Part print with two shaded views. Sizes in mm from the minimum x, y, z corner. A direction names the side the tool comes from. Give positions to 0.01 mm unless a question says otherwise; leave off trailing zeros. Order: outer loops, then holes, each group sorted by start corner. A loop starts at its lowest first (then second) coordinate and runs counter-clockwise, first axis right, second up. Notation, with made-up numbers: (-7.5, 35.5) -> (38.5, 35.5) arc R19 cw to (38.5, 69.5) -> close; hole circle Ø8 at (4, 28). An arc over 180 degrees is marked (long way). Write item = value, one per line. Start each with the question number.
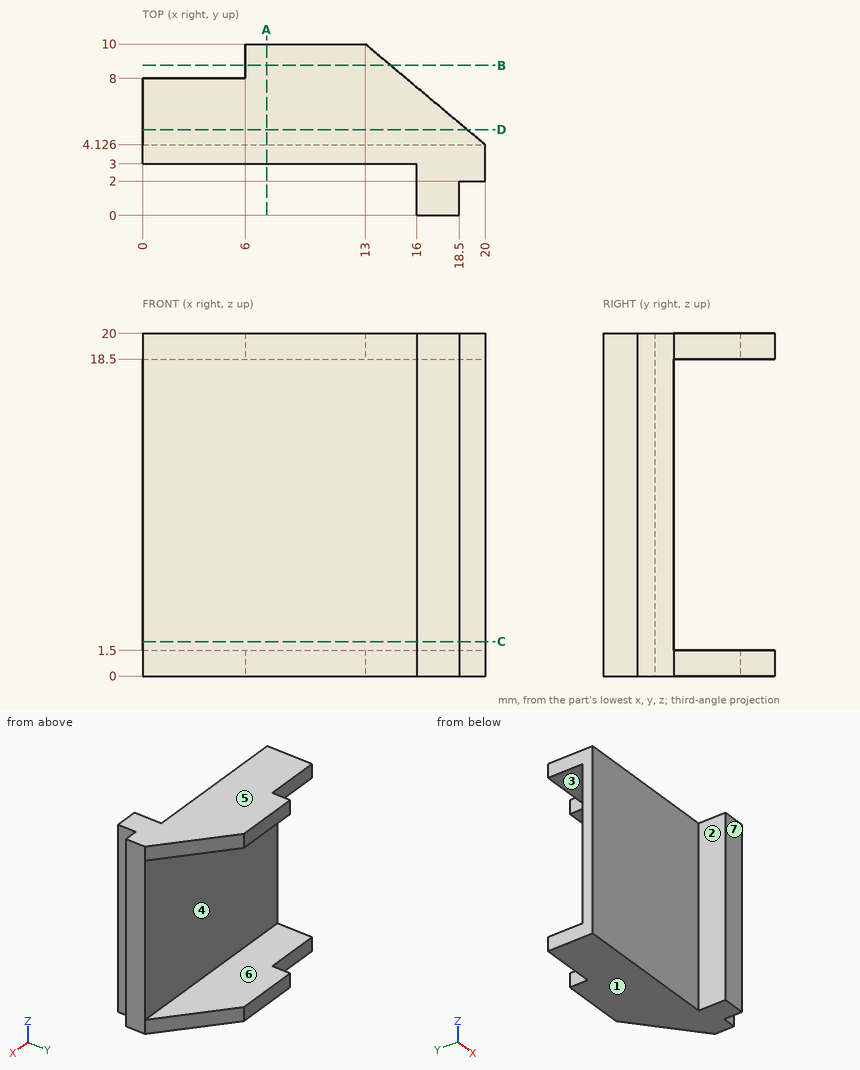
(1) Cut at C-C, the plane z = 2. Give the cut face in (x, y).
(2) 3-axis set-ups, long thin cutter, end or side, ignore diameter. For the marked faces 1, 2 and 3: which of +Z, -Z, +X, -X, +Y, -Y reach the whole face in a straight line?
(3) Cut at B-B, the plane y = 8.75. Give the cut face in (x, z).
(4) Flat gauge pins, fed straight in: P1, Ø0.8, axis at x = 19, z = 12.5, coming from the -Y side; P2, Ø2, axis at x = 13.5, z = 8.5, coming from the +Y side; P3, Ø3, axis at y = 8.5, z = 4.5, coming from the +X side; P4, Ø1.2, axis at y = 9, z = 19, coming from the -X side. Where does each tip first touch, or does it go through?
(5) Wall check: line 1 (Z direction, x = 8, y = 6.75); line 2 (Y direction, x = 4.5, z = 3.75); line 3 (X direction, y = 1, z = 15). Give the ranges that are in metal, low to high. Write a range as [from, to].
(6) Cut at A-A, the plane x = 7.25. Give the cut face in (y, z).
(7) Mould opens along Z. For the marked faces 4, 5, 6 and 7 say: released by +Z, released by -Z, zero draft, split by the parting line, or undercut.
(8) Cut at D-D, the plane y = 5. Give the cut face in (x, z).
Results:
q1.outline = (0, 3) -> (16, 3) -> (16, 0) -> (18.5, 0) -> (18.5, 2) -> (20, 2) -> (20, 4.13) -> (0, 4.13) -> close
q2.face_1 = -Z, +X, -X, +Y, -Y
q2.face_2 = +Z, -Z, -X, -Y
q2.face_3 = +X, -X, +Y
q3.outline = (6, 0) -> (14.49, 0) -> (14.49, 1.5) -> (6, 1.5) -> close; (6, 18.5) -> (14.49, 18.5) -> (14.49, 20) -> (6, 20) -> close
q4.P1 = 2
q4.P2 = 4.13
q4.P3 = through
q4.P4 = 6
q5.line_1 = [0, 1.5], [18.5, 20]
q5.line_2 = [3, 4.13]
q5.line_3 = [16, 18.5]
q6.outline = (3, 0) -> (10, 0) -> (10, 1.5) -> (4.13, 1.5) -> (4.13, 18.5) -> (10, 18.5) -> (10, 20) -> (3, 20) -> close
q7.face_4 = undercut
q7.face_5 = released by +Z
q7.face_6 = undercut
q7.face_7 = zero draft
q8.outline = (0, 0) -> (18.96, 0) -> (18.96, 1.5) -> (0, 1.5) -> close; (0, 18.5) -> (18.96, 18.5) -> (18.96, 20) -> (0, 20) -> close
